The listing builds one solid part. Answer for the finished solid, in the listing's coordinates (mm). Coordinates: 2 decimals unless noted, no trailing zeros. Answer in a Markdown table with one row per item.
```python
from build123d import *

# Parameters (mm, degrees)
SKETCH1_W           = 160.31
SKETCH1_H           = 20
BOSS_EXTRUDE1_DEPTH = 2
CUT_EXTRUDE1_REACH  = 82.801
SKETCH2_R           = 1.4224


with BuildPart() as part:
    # Sketch1 → Boss-Extrude1 (new body)
    with BuildSketch(Plane.XY):
        Rectangle(SKETCH1_W, SKETCH1_H)
    extrude(amount=BOSS_EXTRUDE1_DEPTH)

    # Sketch2 → Cut-Extrude1 (cut, up to next)
    with BuildSketch(Plane.XY.offset(2), mode=Mode.PRIVATE) as cut_extrude1_sk1:
        with Locations((-73.805, 6.825)):
            Circle(SKETCH2_R)
    cut_extrude1_tool1 = extrude(cut_extrude1_sk1.sketch, amount=-CUT_EXTRUDE1_REACH, mode=Mode.PRIVATE) & part.part
    # Sketch2 → Cut-Extrude1 (cut, up to next)
    with BuildSketch(Plane.XY.offset(2), mode=Mode.PRIVATE) as cut_extrude1_sk2:
        with Locations((-73.805, 0.475)):
            Circle(SKETCH2_R)
    cut_extrude1_tool2 = extrude(cut_extrude1_sk2.sketch, amount=-CUT_EXTRUDE1_REACH, mode=Mode.PRIVATE) & part.part
    # Sketch2 → Cut-Extrude1 (cut, up to next)
    with BuildSketch(Plane.XY.offset(2), mode=Mode.PRIVATE) as cut_extrude1_sk3:
        with Locations((-73.805, -5.875)):
            Circle(SKETCH2_R)
    cut_extrude1_tool3 = extrude(cut_extrude1_sk3.sketch, amount=-CUT_EXTRUDE1_REACH, mode=Mode.PRIVATE) & part.part
    # Sketch2 → Cut-Extrude1 (cut, up to next)
    with BuildSketch(Plane.XY.offset(2), mode=Mode.PRIVATE) as cut_extrude1_sk4:
        with Locations((75.155, 5)):
            Circle(SKETCH2_R)
    cut_extrude1_tool4 = extrude(cut_extrude1_sk4.sketch, amount=-CUT_EXTRUDE1_REACH, mode=Mode.PRIVATE) & part.part
    # Sketch2 → Cut-Extrude1 (cut, up to next)
    with BuildSketch(Plane.XY.offset(2), mode=Mode.PRIVATE) as cut_extrude1_sk5:
        with Locations((55.155, 5)):
            Circle(SKETCH2_R)
    cut_extrude1_tool5 = extrude(cut_extrude1_sk5.sketch, amount=-CUT_EXTRUDE1_REACH, mode=Mode.PRIVATE) & part.part
    # Sketch2 → Cut-Extrude1 (cut, up to next)
    with BuildSketch(Plane.XY.offset(2), mode=Mode.PRIVATE) as cut_extrude1_sk6:
        with Locations((55.155, -5)):
            Circle(SKETCH2_R)
    cut_extrude1_tool6 = extrude(cut_extrude1_sk6.sketch, amount=-CUT_EXTRUDE1_REACH, mode=Mode.PRIVATE) & part.part
    # Sketch2 → Cut-Extrude1 (cut, up to next)
    with BuildSketch(Plane.XY.offset(2), mode=Mode.PRIVATE) as cut_extrude1_sk7:
        with Locations((75.155, -5)):
            Circle(SKETCH2_R)
    cut_extrude1_tool7 = extrude(cut_extrude1_sk7.sketch, amount=-CUT_EXTRUDE1_REACH, mode=Mode.PRIVATE) & part.part
    add(cut_extrude1_tool1.solids().sort_by_distance((-73.805, 6.825, 2))[0], mode=Mode.SUBTRACT)
    add(cut_extrude1_tool2.solids().sort_by_distance((-73.805, 0.475, 2))[0], mode=Mode.SUBTRACT)
    add(cut_extrude1_tool3.solids().sort_by_distance((-73.805, -5.875, 2))[0], mode=Mode.SUBTRACT)
    add(cut_extrude1_tool4.solids().sort_by_distance((75.155, 5, 2))[0], mode=Mode.SUBTRACT)
    add(cut_extrude1_tool5.solids().sort_by_distance((55.155, 5, 2))[0], mode=Mode.SUBTRACT)
    add(cut_extrude1_tool6.solids().sort_by_distance((55.155, -5, 2))[0], mode=Mode.SUBTRACT)
    add(cut_extrude1_tool7.solids().sort_by_distance((75.155, -5, 2))[0], mode=Mode.SUBTRACT)


solid = part.part
```
(1) Find the intervals of material crossed by line 1 along X through (y, z) = (-6.75, 1.15) (3 decimals); line 2 along X through (y, z) = (0, 0.7) (3 decimals), in increasing order. Write a range as from..to.
Check values:
| item | result |
|---|---|
| line 1 | -80.155..-74.926, -72.684..80.155 |
| line 2 | -80.155..-75.146, -72.464..80.155 |
(2) A flat-ended cylindrical pin translates along its axis: pin 1 (2.5 mm diameter, centred on x = 75.155, y = 5, fed in from -Z). Find the tip coordinate at first contact, or state that the pin passes through.
Check values:
| item | result |
|---|---|
| pin 1 | through |
(3) For a pull along X with two mould halves and no side action, classify faces 1 (the cylindrical face through (54.107, 5.961, 1.014)), 2 (the cylindrical face through (-72.49, -0.07, 1.01)), 3 (the flat face through (-1, 0, 0)) as released by +X, released by -X, zero draft, split by the parting line, or undercut.
Check values:
| item | result |
|---|---|
| face 1 | undercut |
| face 2 | undercut |
| face 3 | zero draft |
